Study the drawing (mm; zero at the part's minimum x, y, z) and answer. A direction names the side the tool comes from. Coordinates: 2 decimals unless noted, no trailing zeros. Write each loop counter-clockwise with the first axis right and the second up, starting at its lowest first coordinate (ties: lowest second). Pieces come first, ordered by that corner, then holes. Notation, with made-up numbers: M -35.75,-20.5 L 8.25,-20.5 A14 ccw 8.25,3.5 Z; hole C -33,77.5 d1. An arc over 180 degrees is marked long. Answer as CSV lines item,"result". Start each with the question number.
(1) The mould has two halves that part along X. Classify the marked faces 1, 2 and 3: released by +X, released by -X, zero draft, split by the parting line, or undercut.
(2) A cutting plane is placed at D-D on y = 14. Give the vertices of the cut face in (x, z) (1 decimal).
(3) A cutting plane is placed at C-C on x = 1.5. Give the vertices of the cut face in (y, z).
(4) A cutting plane is placed at A-A on y = 4. Give the vertices of the cut face in (x, z).
(5) Find the intervals of material crossed by L1, parallel to X at y = 16.25, z = 1.75; L2, parallel to X at y = 8.75, z = 5.25; L3, parallel to Y at x = 5, z = 6, in increasing order. Write a range as [from, to].
(6) For the marked faces 4, 5, 6 and 7, determine the directions among +Z, -Z, +X, -X, +Y, -Y from which every point of the face is accessible in a straight line to the end or side of a thin tool.
(7) Flat-ended cylindrical pins translate along their axes: P1, Ø2.5, axis at y = 10.922, z = 4.064, coming from the +X side; P2, Ø2.5, axis at y = 12.5, z = 3.5, coming from the +X side; P3, Ø2.5, axis at x = 12.5, z = 4.5, coming from the +Y side; P4, Ø0.6, axis at x = 15.5, z = 5, coming from the +Y side. Find the tip coordinate at first contact, or state that the pin passes through.
(8) A cutting plane is placed at B-B on z = 6.75. Give the vertices of the cut face in (x, y), then the cut area to 3 significant figures.
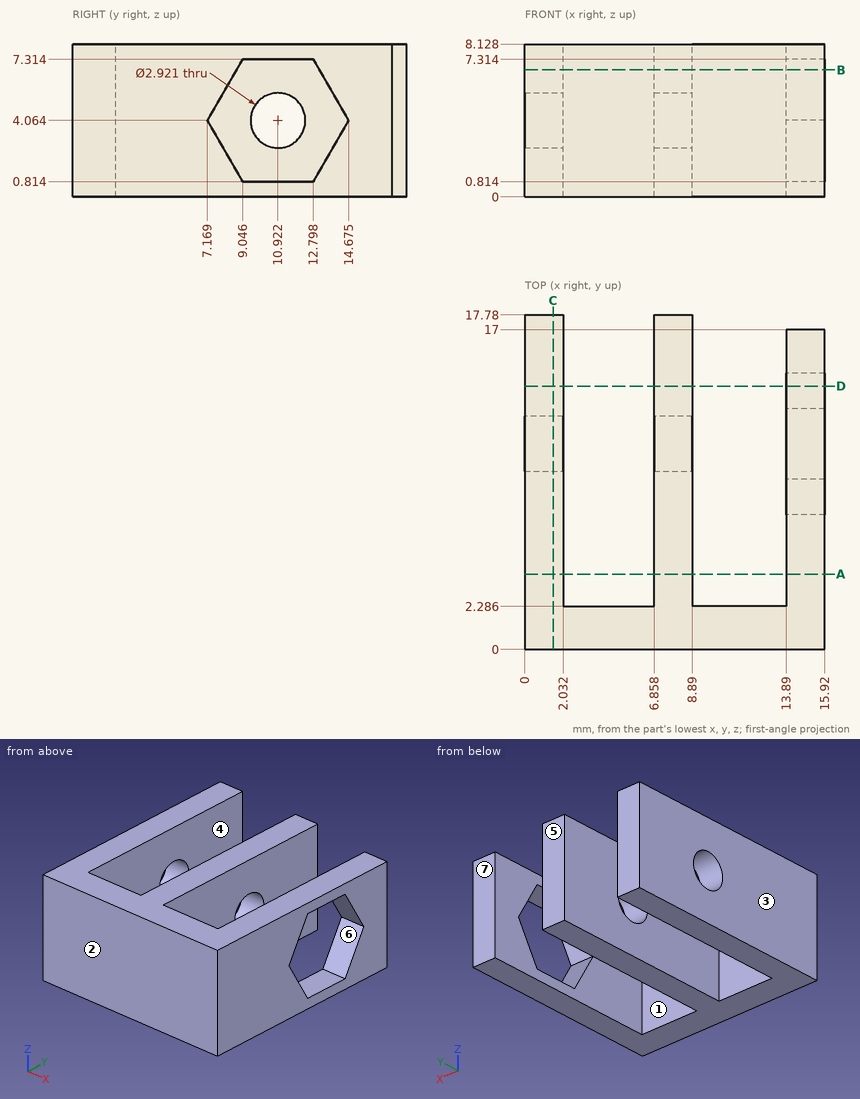
Here are the results:
1,face 1,"undercut"
1,face 2,"zero draft"
1,face 3,"released by -X"
2,outline,"M 0,0 L 2,0 L 2,8.1 L 0,8.1 Z; M 6.9,0 L 8.9,0 L 8.9,8.1 L 6.9,8.1 Z; M 13.9,0 L 15.9,0 L 15.9,2.9 L 13.9,2.9 Z; M 13.9,5.2 L 15.9,5.2 L 15.9,8.1 L 13.9,8.1 Z"
3,outline,"M 0,0 L 17.78,0 L 17.78,8.13 L 0,8.13 Z; hole C 10.92,4.06 d2.92"
4,outline,"M 0,0 L 2.03,0 L 2.03,8.13 L 0,8.13 Z; M 6.86,0 L 8.89,0 L 8.89,8.13 L 6.86,8.13 Z; M 13.89,0 L 15.92,0 L 15.92,8.13 L 13.89,8.13 Z"
5,L1,"x = [0, 2.03], [6.86, 8.89], [13.89, 15.92]"
5,L2,"x = [0, 2.03], [6.86, 8.89]"
5,L3,"y = [0, 2.29]"
6,face 4,"+Z, -Z, +Y"
6,face 5,"+Z, -Z, +X, -X, +Y"
6,face 6,"+X"
6,face 7,"+Z, -Z, +X, +Y"
7,P1,"passes through"
7,P2,"stops at x = 8.89"
7,P3,"stops at y = 2.29"
7,P4,"stops at y = 17"
8,outline,"M 0,0 L 15.92,0 L 15.92,8.72 L 13.89,8.72 L 13.89,2.29 L 8.89,2.29 L 8.89,17.78 L 6.86,17.78 L 6.86,2.29 L 2.03,2.29 L 2.03,17.78 L 0,17.78 Z; M 13.89,13.12 L 15.92,13.12 L 15.92,17 L 13.89,17 Z"
8,area,"120 mm^2"
